Part model, mm, in its own coordinate system. Round coordinates to 2 decimals unless told otherwise and drop trailing zeros. Write each loop counter-clockwise with the first axis right and the second up, starting at its lowest first coordinate (ties: lowest second). Pieces come first, ordered by that corner, then holes.
```python
from build123d import *

# Parameters (mm, degrees)
SKETCH1_R           = 5
SKETCH1_R_2         = 11
BOSS_EXTRUDE1_DEPTH = 8


with BuildPart() as part:
    # Sketch1 → Boss-Extrude1 (new body)
    with BuildSketch(Plane.XY):
        with BuildLine():
            Line((-22, -22), (22, -22))
            ThreePointArc((22, -22), (25.535533906, -20.535533906), (27, -17))
            Line((27, -17), (27, 17))
            Line((27, 17), (-27, 17))
            Line((-27, 17), (-27, -17))
            ThreePointArc((-27, -17), (-25.535533906, -20.535533906), (-22, -22))
        make_face()
        with Locations((-19, 0)):
            Circle(SKETCH1_R, mode=Mode.SUBTRACT)
        with Locations((19, 0)):
            Circle(SKETCH1_R, mode=Mode.SUBTRACT)
        Circle(SKETCH1_R_2, mode=Mode.SUBTRACT)
    extrude(amount=BOSS_EXTRUDE1_DEPTH)


solid = part.part
```
Q1. Cut at C-C on z = 4.5. Write the cut outline in (x, y), plus the area to 3 significant figures.
Values follow:
outline: (-27, -17) arc R5 ccw to (-22, -22) - (22, -22) arc R5 ccw to (27, -17) - (27, 17) - (-27, 17) - close; hole circle Ø10 at (-19, 0); hole circle Ø22 at (0, 0); hole circle Ø10 at (19, 0)
area: 1,560 mm2
Q2. Wall check: L1, parallel to Y at x = 0, z = 6.75; L2, parallel to Y at x = 19, z = 3.25; L3, parallel to X at y = -3.5, z = 5.25. Give the ranges that are in metal, low to high.
Values follow:
L1: y = -22 to -11, 11 to 17
L2: y = -22 to -5, 5 to 17
L3: x = -27 to -22.57, -15.43 to -10.43, 10.43 to 15.43, 22.57 to 27
Q3. Cut at A-A on x = 0. Write the cut outline in (y, z).
Values follow:
outline: (-22, 0) - (-11, 0) - (-11, 8) - (-22, 8) - close; (11, 0) - (17, 0) - (17, 8) - (11, 8) - close
Q4. Cut at D-D on y = -9. Write the cut outline in (x, z), plus the area to 3 significant figures.
Values follow:
outline: (-27, 0) - (-6.32, 0) - (-6.32, 8) - (-27, 8) - close; (6.32, 0) - (27, 0) - (27, 8) - (6.32, 8) - close
area: 331 mm2
Q5. Mould opens along Y. For faces 1 (the flat face through (6, -11, 0)), 2 (the flat face through (0, -22, 4)), 3 (the flat face through (0, 17, 4)), 4 (the cylindrical face through (14, 0, 4)) say: +Y half, -Y half, draft (parallel to the pull), parting line (faces both ways), or undercut.
Values follow:
face 1: draft
face 2: -Y half
face 3: +Y half
face 4: undercut
Q6. Cut at B-B on y = 0. Write the cut outline in (x, z), plus the area to 3 significant figures.
Values follow:
outline: (-27, 0) - (-24, 0) - (-24, 8) - (-27, 8) - close; (-14, 0) - (-11, 0) - (-11, 8) - (-14, 8) - close; (11, 0) - (14, 0) - (14, 8) - (11, 8) - close; (24, 0) - (27, 0) - (27, 8) - (24, 8) - close
area: 96.0 mm2
